Source: CAD feature listing. Evaluate the final solid. Frame: model axes, mm. Face numbers are marked on the shaded views. A direction names the side the tool comes from. Give positions to 0.01 mm unless a question says otherwise; leave off trailing zeros. Order: outer loops, then holes, each group sorted by start corner. A loop starts at its lowest first (then second) coordinate and runs counter-clockwise, first axis right, second up. Notation, with made-up numbers: (89, 48) -> (104, 48) arc R19 cw to (104, 83) -> close; hole circle Ø6 at (-21, 22). An arc over 180 degrees is marked (long way). Use CSV: the item, a comma, the result in double quotes.
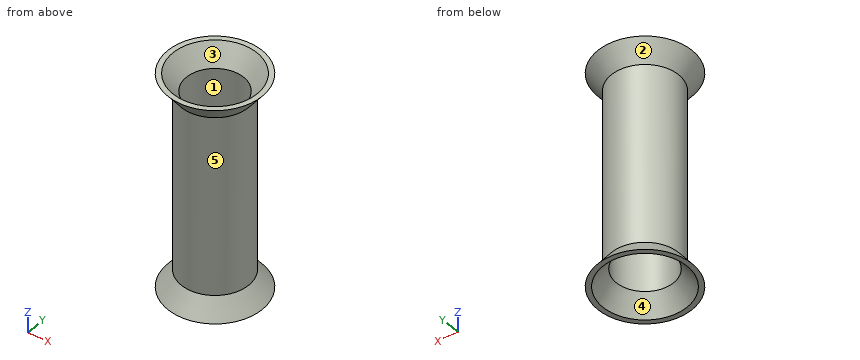
```python
from build123d import *

# Parameters (mm, degrees)
SKETCH2_R           = 4.7625
SKETCH2_R_2         = 4.0513
BOSS_EXTRUDE1_DEPTH = 12.7
SKETCH4_R           = 4.7625
BOSS_EXTRUDE2_DEPTH = 2.54
BOSS_EXTRUDE2_DRAFT = -37


# Read off the part's stored shape, not the designer's step: Mirror1
with BuildPart() as part:
    # Sketch2 → Boss-Extrude1 (new, symmetric)
    with BuildSketch(Plane.XY):
        Circle(SKETCH2_R)
        Circle(SKETCH2_R_2, mode=Mode.SUBTRACT)
    extrude(amount=BOSS_EXTRUDE1_DEPTH, both=True)


with BuildPart() as boss_extrude2_tool:
    # Sketch4 → Boss-Extrude2 (with draft: the straight prism first)
    with BuildSketch(Plane(origin=(0, 0, -12.7), x_dir=(-1, 0, 0), z_dir=(0, 0, -1))):
        Circle(SKETCH4_R)
    extrude(amount=BOSS_EXTRUDE2_DEPTH)
    # Boss-Extrude2: the draft: its side faces are tilted about the plane it starts from
    boss_extrude2_sides = [boss_extrude2_tool.faces().sort_by_distance(p)[0] for p in [
        (4.7625, 0, -13.97),
    ]]
    draft(boss_extrude2_sides, Plane(origin=(0, 0, -12.7), x_dir=(-1, 0, 0), z_dir=(0, 0, -1)), BOSS_EXTRUDE2_DRAFT)


with BuildPart() as part_1:
    add(part.part)

    # Boss-Extrude2: add boss_extrude2_tool
    add(boss_extrude2_tool.part)

    # Cut-Extrude2 cone 1 section (on through the dimple's axis) → Cut-Extrude2 (revolve, cut)
    with BuildSketch(Plane(origin=(0, 0, -15.24), x_dir=(0, 1, 0), z_dir=(1, 0, 0))):
        Polygon((0, 0), (5.965327287, 0), (0, 7.916256686), align=None)
    revolve(axis=Axis((0, 0, -15.24), (0, 0, 1)), mode=Mode.SUBTRACT)

    # Mirror1 outline → Mirror1 (revolve)
    with BuildSketch(Plane.XZ):
        Polygon((4.0513, 12.7), (4.7625, 12.7), (6.676527287, 15.24), (5.965327287, 15.24), align=None)
    revolve(axis=Axis((0, 0, 0), (0, 0, 1)))


solid = part_1.part
```
1. Access query for the marked faces 1 and 2. Directions: +Z, -Z, +X, -X, +Y, -Y. A direction counts if a zero-diameter tool reaches every point of the face in a straight line with its end or side. Return the directions, or none.
Answer below:
face 1,"+Z, -Z"
face 2,"none"
2. Pin query (flat end, axial travel): P1, Ø6, axis at y = 4.5, z = 4.5, coming from the +X side; P2, Ø4, axis at y = 2.5, z = 3, coming from the +X side; P3, Ø6, axis at x = 0.5, y = -4.5, coming from the -Z side; P4, Ø3, axis at y = -1.5, z = 8, coming from the +X side. Return the tip coordinate at first contact, or that it passes through.
Answer below:
P1,"stops at x = 4.52"
P2,"stops at x = 4.74"
P3,"stops at z = -15.24"
P4,"stops at x = 4.76"
3. Section query A-A on y = 0. Return loops of the section in (x, z), plus the area to 3 significant figures.
Answer below:
outline,"(-6.68, -15.24) -> (-5.97, -15.24) -> (-4.05, -12.7) -> (-4.05, 12.7) -> (-5.97, 15.24) -> (-6.68, 15.24) -> (-4.76, 12.7) -> (-4.76, -12.7) -> close; (4.05, -12.7) -> (5.97, -15.24) -> (6.68, -15.24) -> (4.76, -12.7) -> (4.76, 12.7) -> (6.68, 15.24) -> (5.97, 15.24) -> (4.05, 12.7) -> close"
area,"43.4 mm²"
4. Mould query, pull axis Z, two halves, no side actions, for the marked faces 3, 4 and 5. Classes: released by +Z, released by -Z, zero draft, split by the parting line, or undercut.
Answer below:
face 3,"released by +Z"
face 4,"released by -Z"
face 5,"undercut"
5. Section query C-C on z = -4. Return loops of the section in (x, y) (1 decimal).
Answer below:
outline,"circle Ø9.5 at (0, 0); hole circle Ø8.1 at (0, 0)"
6. Ray query, line 1 along Y through (x, z) = (0.25, -10.5); line 2 along X through (y, z) = (0, 4.75). Return the intervals inside material, ascending.
Answer below:
line 1,"y = -4.76 to -4.04, 4.04 to 4.76"
line 2,"x = -4.76 to -4.05, 4.05 to 4.76"
